Build history of the part. All positions in model axes, mm. Give positions to 0.01 mm unless a question says otherwise; leave off trailing zeros. Order: outer loops, then holes, each group sorted by start corner. A loop starts at its lowest first (then second) coordinate and runs counter-clockwise, first axis right, second up. Notation, with made-up numbers: (48, 44) - (94, 44) arc R24 ccw to (94, 55) - close; hole circle Ø7 at (7.5, 43). An arc over 180 degrees is marked (long way). Use a Markdown table: item, result.
from build123d import *

# Parameters (mm, degrees)
BOSS_EXTRUDE1_OUTLINE_R   = 2.75
BOSS_EXTRUDE1_OUTLINE_R_2 = 5
BOSS_EXTRUDE1_OUTLINE_R_3 = 2.499999993
BOSS_EXTRUDE1_OUTLINE_R_4 = 3
BOSS_EXTRUDE1_OUTLINE_R_5 = 6
BOSS_EXTRUDE1_DEPTH       = 5
CUT_EXTRUDE1_DEPTH        = 5


# Read off the part's stored shape, not the designer's step: Boss-Extrude1
with BuildPart() as part:
    # Boss-Extrude1 outline → Boss-Extrude1 (new body)
    with BuildSketch(Plane.XY):
        with BuildLine():
            ThreePointArc((56.677553307, -117.080446425), (63.779903671, -109.786095566), (66.371177049, -99.940475351))
            Line((66.371177049, -99.940475351), (66.371177049, 7.470187014))
            ThreePointArc((66.371177049, 7.470187014), (60.513312673, 21.612322638), (46.371177049, 27.470187014))
            Line((46.371177049, 27.470187014), (-56.688822951, 27.470187014))
            ThreePointArc((-56.688822951, 27.470187014), (-59.277013402, 27.810928751), (-61.688822951, 28.809932976))
            Line((-61.688822951, 28.809932976), (-314.412271613, 174.719884092))
            ThreePointArc((-314.412271613, 174.719884092), (-322.213114889, 175.659384058), (-328.284834714, 170.672397556))
            ThreePointArc((-328.284834714, 170.672397556), (-369.976805992, 4.142827069), (-332.024261256, -163.278565422))
            Line((-332.024261256, -163.278565422), (-20.152013506, -163.278565422))
            Line((-20.152013506, -163.278565422), (56.677553307, -117.080446425))
        make_face()
        with Locations((-318.548901543, -117.417406357)):
            Circle(BOSS_EXTRUDE1_OUTLINE_R, mode=Mode.SUBTRACT)
        with Locations((-323.727269541, -102.278565422)):
            Circle(BOSS_EXTRUDE1_OUTLINE_R_2, mode=Mode.SUBTRACT)
        with Locations((-328.90563754, -87.139724486)):
            Circle(BOSS_EXTRUDE1_OUTLINE_R, mode=Mode.SUBTRACT)
        with Locations((-260.152013506, -143.278565422)):
            Circle(BOSS_EXTRUDE1_OUTLINE_R_3, mode=Mode.SUBTRACT)
        with Locations((-200.152013506, -143.278565422)):
            Circle(BOSS_EXTRUDE1_OUTLINE_R_3, mode=Mode.SUBTRACT)
        with Locations((-339.2241853, -13.682181731)):
            Circle(BOSS_EXTRUDE1_OUTLINE_R, mode=Mode.SUBTRACT)
        with Locations((-339.492103151, 2.315574988)):
            Circle(BOSS_EXTRUDE1_OUTLINE_R_2, mode=Mode.SUBTRACT)
        with Locations((-140.152013506, -143.278565422)):
            Circle(BOSS_EXTRUDE1_OUTLINE_R_3, mode=Mode.SUBTRACT)
        with Locations((-80.152013506, -143.278565422)):
            Circle(BOSS_EXTRUDE1_OUTLINE_R_3, mode=Mode.SUBTRACT)
        with Locations((-24, 0)):
            Circle(BOSS_EXTRUDE1_OUTLINE_R_4, mode=Mode.SUBTRACT)
        with Locations((1.6e-08, 2e-09)):
            Circle(BOSS_EXTRUDE1_OUTLINE_R_5, mode=Mode.SUBTRACT)
        with Locations((24, 0)):
            Circle(BOSS_EXTRUDE1_OUTLINE_R_4, mode=Mode.SUBTRACT)
        with Locations((-339.760021002, 18.313331706)):
            Circle(BOSS_EXTRUDE1_OUTLINE_R, mode=Mode.SUBTRACT)
        with Locations((-319.497069854, 114.812335336)):
            Circle(BOSS_EXTRUDE1_OUTLINE_R, mode=Mode.SUBTRACT)
        with Locations((-313.732870505, 129.737951098)):
            Circle(BOSS_EXTRUDE1_OUTLINE_R_2, mode=Mode.SUBTRACT)
        with Locations((-307.968671157, 144.66356686)):
            Circle(BOSS_EXTRUDE1_OUTLINE_R, mode=Mode.SUBTRACT)
    extrude(amount=BOSS_EXTRUDE1_DEPTH)

    # Sketch2 → Cut-Extrude1 (cut)
    with BuildSketch(Plane.XY.offset(5)):
        Polygon((-155, -7), (-170, 18.980762114), (-200, 18.980762114), (-215, -7), (-200, -32.980762114), (-170, -32.980762114), align=None)
        Polygon((-103.038475773, -37), (-118.038475773, -11.019237886), (-148.038475773, -11.019237886), (-163.038475773, -37), (-148.038475773, -62.980762114), (-118.038475773, -62.980762114), align=None)
        Polygon((-215, -127), (-155, -127), (-170, -101.019237886), (-200, -101.019237886), align=None)
        Polygon((-111.076951546, -127), (-51.076951546, -127), (-66.076951546, -101.019237886), (-96.076951546, -101.019237886), align=None)
        Polygon((-51.076951546, -67), (-66.076951546, -41.019237886), (-96.076951546, -41.019237886), (-111.076951546, -67), (-96.076951546, -92.980762114), (-66.076951546, -92.980762114), align=None)
        Polygon((-118.038475773, -2.980762114), (-103.038475773, 23), (-118.038475773, 48.980762114), (-148.038475773, 48.980762114), (-163.038475773, 23), (-148.038475773, -2.980762114), align=None)
        Polygon((-258.923048454, 53), (-273.923048454, 78.980762114), (-303.923048454, 78.980762114), (-318.923048454, 53), (-303.923048454, 27.019237886), (-273.923048454, 27.019237886), align=None)
        Polygon((-206.961524227, 23), (-221.961524227, 48.980762114), (-251.961524227, 48.980762114), (-266.961524227, 23), (-251.961524227, -2.980762114), (-221.961524227, -2.980762114), align=None)
        Polygon((-221.961524227, 57.019237886), (-206.961524227, 83), (-221.961524227, 108.980762114), (-251.961524227, 108.980762114), (-266.961524227, 83), (-251.961524227, 57.019237886), align=None)
        Polygon((-170, 27.019237886), (-155, 53), (-170, 78.980762114), (-200, 78.980762114), (-215, 53), (-200, 27.019237886), align=None)
        Polygon((-66.076951546, -32.980762114), (-51.076951546, -7), (-66.076951546, 18.980762114), (-96.076951546, 18.980762114), (-111.076951546, -7), (-96.076951546, -32.980762114), align=None)
        Polygon((-103.038475773, -97), (-118.038475773, -71.019237886), (-148.038475773, -71.019237886), (-163.038475773, -97), (-148.038475773, -122.980762114), (-118.038475773, -122.980762114), align=None)
        Polygon((-170, -41.019237886), (-200, -41.019237886), (-215, -67), (-200, -92.980762114), (-170, -92.980762114), (-155, -67), align=None)
        Polygon((-273.923048454, -32.980762114), (-258.923048454, -7), (-273.923048454, 18.980762114), (-303.923048454, 18.980762114), (-318.923048454, -7), (-303.923048454, -32.980762114), align=None)
        Polygon((-221.961524227, -62.980762114), (-206.961524227, -37), (-221.961524227, -11.019237886), (-251.961524227, -11.019237886), (-266.961524227, -37), (-251.961524227, -62.980762114), align=None)
        Polygon((-273.923048454, 87.019237886), (-258.923048454, 113), (-273.923048454, 138.980762114), (-303.923048454, 87.019237886), align=None)
        Polygon((-303.923048454, -92.980762114), (-273.923048454, -92.980762114), (-258.923048454, -67), (-273.923048454, -41.019237886), (-303.923048454, -41.019237886), (-318.923048454, -67), align=None)
        Polygon((-206.961524227, -97), (-221.961524227, -71.019237886), (-251.961524227, -71.019237886), (-266.961524227, -97), (-251.961524227, -122.980762114), (-221.961524227, -122.980762114), align=None)
    extrude(amount=-CUT_EXTRUDE1_DEPTH, mode=Mode.SUBTRACT)


solid = part.part
1) Slice it at A-A (y = 72.5). Write the cut outline in (x, z), and give its area (3 significant figures).
Computed:
| item | result |
|---|---|
| outline | (-362.83, 0) - (-307.66, 0) - (-307.66, 5) - (-362.83, 5) - close; (-270.18, 0) - (-260.9, 0) - (-260.9, 5) - (-270.18, 5) - close; (-213.02, 0) - (-203.74, 0) - (-203.74, 5) - (-213.02, 5) - close; (-166.26, 0) - (-137.36, 0) - (-137.36, 5) - (-166.26, 5) - close |
| area | 513 mm² |
2) Wall check: line 1 (X direction, y = -98, z = 1.4); line 2 (X direction, y = 100, z = 2.6); line 3 (X direction, y = 67, z = 1.3). Give the ranges that are in metal, low to high. Write a range as from..to.
Computed:
| item | result |
|---|---|
| line 1 | x = -356.79..-326.31, -321.14..-266.38, -207.54..-162.46, -103.62..66.37 |
| line 2 | x = -356.23..-296.43, -266.43..-257.15, -216.78..-184.99 |
| line 3 | x = -363.88..-310.84, -267.01..-257.72, -216.2..-206.92, -163.08..-127.84 |
3) Two-plate mould, pull along Y, no slides. Class faces 1 (the cylindrical face through (-369.94, 6.57, 2.46)), 2 (the flat face through (-288.713, 113.364, 2.535)), 3 (the flat face through (17.725, -140.503, 2.465)): +Y half, -Y half, draft (parallel to the pull), parting line (faces both ways), or undercut.
Computed:
| item | result |
|---|---|
| face 1 | parting line |
| face 2 | undercut |
| face 3 | -Y half |
4) Slice it at C-C (z = 3.1). State how many separate pieces and enclosed holes the cut face has, and give its area (3 significant figures).
Computed:
| item | result |
|---|---|
| separate pieces | 1 |
| enclosed holes | 34 |
| area | 64,100 mm² |
5) Slice it at B-B (x = 0). Write the cut outline in (y, z).
Computed:
| item | result |
|---|---|
| outline | (-151.16, 0) - (-6, 0) - (-6, 5) - (-151.16, 5) - close; (6, 0) - (27.47, 0) - (27.47, 5) - (6, 5) - close |
6) Slice it at D-D (y = -134). Write the cut outline in (x, z).
Computed:
| item | result |
|---|---|
| outline | (-344.88, 0) - (28.54, 0) - (28.54, 5) - (-344.88, 5) - close |
7) Pin check, flat tips, straight feed: P1, Ø2.5, axis at x = -241.5, z = 3.5, coming from the +Y side; P2, Ø2, axis at y = 136, z = 1.5, coming from the -X side; P3, Ø6.5, axis at x = -307.97, y = 144.66, coming from the +Z side; P4, Ø2.5, axis at x = -230.5, z = 3, coming from the +Y side. Stop position of each tip, or through.
Computed:
| item | result |
|---|---|
| P1 | stops at y = 133.35 |
| P2 | stops at x = -344.49 |
| P3 | stops at z = 5 |
| P4 | stops at y = 126.99 |
